Check sheet for the modelled part. Datum: model origin and axes. Units: mm. A direction names the side the tool comes from. Round coordinates to 2 decimals unless told otherwise and drop trailing zeros. Order: outer loops, then holes, each group sorted by start corner. A loop starts at its lowest first (then second) coordinate and runs counter-clockwise, first axis right, second up. Notation, with made-up numbers: (53.5, 66.25) -> (108.5, 66.25) arc R20 cw to (108.5, 71.25) -> close; hole circle Ø10 at (-25, 75.25). An arc over 180 degrees is marked (long way). Answer in a Markdown table with one row per item. Add a question column.
1. Draft check along Z on faces 3 (the cylindrical face through (5.921, -1.207, 18.414)), 4 (the flat face through (5, -1, 0)), 5 (the flat face through (0, -1, 8)). Enter one of: +Z half, -Z half, draft (parallel to the pull), parting line (faces both ways), or undercut.
2. Sectioned sample at A-A, the plane y = -0.4. Record the boundary of the cut face in (x, z) (3 decimals), then the cut area to 3 significant figures.
3. Access from +Z, -Z, +X, -X, +Y, -Y to the whole of each face (thin tool, end or side, straight path). Record for faces 1 (the flat face through (27, 0, 16)), 2 (the flat face through (39, -1, 21.494)).
4. Sectioned sample at C-C, the plane x = 49. Record the boundary of the cut face in (y, z).
5. Sectioned sample at B-B, the plane z = 6.5. Record the boundary of the cut face in (x, y).
6. Material ranges on L1, parallel to Z at x = 6.35, y = -1.25; L2, parallel to X at y = -1.15, z = 17; L3, parallel to Z at x = 57, y = -0.5, recorded low to high. Write a range as from..to.
7. Depth check by flat-ended pin: P1, Ø6, axis at x = 52, z = 12, coming from the +Y side; P2, Ø0.7, axis at x = 49.5, y = -1.5, coming from the +Z side. Enter the tip coordinate at first touch or a pass-through.
```python
from build123d import *

# Parameters (mm, degrees)
F1_DEPTH = 2.38125
F2_R     = 3.2981725782
F3_DEPTH = 25.4


# Not quite as in the source:
# - a length typed as a fraction of an inch, garbled in the dataset ("3 / 203.2 mm" for 3/8 in), is restored


with BuildPart() as f1:
    # F0 (on Front) → F1 (new body)
    with BuildSketch(Plane.XZ):
        with BuildLine():
            Line((69.85, 21.4939358442), (6.35, 21.4939358442))
            ThreePointArc((6.35, 21.4939358442), (1.8598719395, 19.6340639047), (0, 15.1439358442))
            Line((0, 15.1439358442), (0, 0))
            Line((0, 0), (9.525, 0))
            Line((9.525, 0), (11.5292743985, 7.4402281731))
            ThreePointArc((11.5292743985, 7.4402281731), (13.0480987591, 10.1527436206), (15.6724793239, 11.8192351874))
            Line((15.6724793239, 11.8192351874), (17.4910178831, 12.4187755322))
            Line((17.4910178831, 12.4187755322), (70.0698060278, 15.1439358442))
            Line((70.0698060278, 15.1439358442), (69.85, 15.1439358442))
            Line((69.85, 15.1439358442), (69.85, 21.4939358442))
        make_face()
        Polygon((69.85, 21.7137452919), (69.85, 21.4939358442), (69.85, 15.1439358442), (70.0698060278, 15.1439358442), (70.0698060278, 21.7137452919), align=None)
    extrude(amount=F1_DEPTH)

    # F2 (on face) → F3 (cut)
    with BuildSketch(Plane.XZ.offset(2.38125)):
        with Locations((6.35, 15.1439358442)):
            Circle(F2_R)
    extrude(amount=-F3_DEPTH, mode=Mode.SUBTRACT)


solid = f1.part
```
Answer key:
| question | item | result |
|---|---|---|
| 1 | face 3 | undercut |
| 1 | face 4 | -Z half |
| 1 | face 5 | draft |
| 2 | outline | (0, 0) -> (9.525, 0) -> (11.529, 7.44) arc R6.35 cw to (15.672, 11.819) -> (17.491, 12.419) -> (70.07, 15.144) -> (70.07, 21.714) -> (69.85, 21.714) -> (69.85, 21.494) -> (6.35, 21.494) arc R6.35 ccw to (0, 15.144) -> close; hole circle Ø6.596 at (6.35, 15.144) |
| 2 | area | 666 mm² |
| 3 | face 1 | +Z, -Z, +X, -X, +Y |
| 3 | face 2 | +Z, -X, +Y, -Y |
| 4 | outline | (-2.38, 14.05) -> (0, 14.05) -> (0, 21.49) -> (-2.38, 21.49) -> close |
| 5 | outline | (0, -2.38) -> (11.28, -2.38) -> (11.28, 0) -> (0, 0) -> close |
| 6 | L1 | z = 0..11.85, 18.44..21.49 |
| 6 | L2 | x = 0.28..3.62, 9.08..70.07 |
| 6 | L3 | z = 14.47..21.49 |
| 7 | P1 | stops at y = 0 |
| 7 | P2 | stops at z = 21.49 |
